Read the model definition and answer for the solid it produces. Units are mm, in the model's axes. A direction names the side the tool comes from. Give positions to 0.01 mm unless a question says otherwise; leave off trailing zeros. Write each loop counter-clockwise with the first axis right and the second up, starting at its lowest first coordinate (ties: lowest second). Pieces come first, ordered by that corner, then holes. Notation, with made-up numbers: (31.25, 66.5) - (44.25, 66.5) arc R13 cw to (44.25, 76.5) - close; hole circle Ø8 at (41, -36.75). An arc over 180 degrees is marked (long way). Answer as CSV lines item,"result".
```python
from build123d import *

# Parameters (mm, degrees)
ESBO_O2_W                = 28
ESBO_O2_H                = 34.43
RESSALTO_EXTRUS_O1_DEPTH = 3
FILETE1_R                = 3
RESSALTO_EXTRUS_O2_START = -1.5
RESSALTO_EXTRUS_O2_DEPTH = 1.5
ESBO_O5_W                = 28
ESBO_O5_H                = 3
RESSALTO_EXTRUS_O3_DEPTH = 20
ESBO_O6_R                = 2.5
CORTE_EXTRUS_O1_DEPTH    = 10
FILETE2_R                = 3
RESSALTO_EXTRUS_O4_DEPTH = 1.5
CHANFRO1_SIZE            = 1.5
CHANFRO2_SIZE            = 1.5
ESBO_O8_R                = 4
CORTE_EXTRUS_O2_DEPTH    = 0.5
CHANFRO3_SIZE            = 5
ESBO_O9_W                = 3
ESBO_O9_H                = 31.43
RESSALTO_EXTRUS_O5_DEPTH = 0.5
CHANFRO4_SIZE            = 0.5


with BuildPart() as part:
    # Esboço2 → Ressalto-extrusão1 (new body)
    with BuildSketch(Plane.XY):
        with Locations((0.050363351, 1.373235294)):
            Rectangle(ESBO_O2_W, ESBO_O2_H)
        with BuildLine():
            Line((8.050363351, 14.888235294), (-7.949636649, 14.888235294))
            ThreePointArc((-7.949636649, 14.888235294), (-9.575982246, 14.214580891), (-10.249636649, 12.588235294))
            Line((-10.249636649, 12.588235294), (-10.249636649, -7.411764706))
            ThreePointArc((-10.249636649, -7.411764706), (-9.575982246, -9.038110303), (-7.949636649, -9.711764706))
            Line((-7.949636649, -9.711764706), (-3.749636649, -9.711764706))
            Line((-3.749636649, -9.711764706), (-3.749636649, -11.711764706))
            Line((-3.749636649, -11.711764706), (3.850363351, -11.711764706))
            Line((3.850363351, -11.711764706), (3.850363351, -9.711764706))
            Line((3.850363351, -9.711764706), (8.050363351, -9.711764706))
            ThreePointArc((8.050363351, -9.711764706), (9.676708947, -9.038110303), (10.350363351, -7.411764706))
            Line((10.350363351, -7.411764706), (10.350363351, 12.588235294))
            ThreePointArc((10.350363351, 12.588235294), (9.676708947, 14.214580891), (8.050363351, 14.888235294))
        make_face(mode=Mode.SUBTRACT)
    extrude(amount=RESSALTO_EXTRUS_O1_DEPTH)

    # Filete1
    filete1_edges = [part.edges().sort_by_distance(p)[0] for p in [
        (-13.949636649, 18.588235294, 1.5),
        (14.050363351, 18.588235294, 1.5),
    ]]
    fillet(filete1_edges, radius=FILETE1_R)

    # Esboço3 → Ressalto-extrusão2 (add)
    with BuildSketch(Plane(origin=(0, 0, 0), x_dir=(-1, 0, 0), z_dir=(0, 0, -1)).offset(RESSALTO_EXTRUS_O2_START)):
        with BuildLine():
            Line((13.949636649, 15.588235294), (13.949636649, -15.841764706))
            Line((13.949636649, -15.841764706), (-14.050363351, -15.841764706))
            Line((-14.050363351, -15.841764706), (-14.050363351, 15.588235294))
            ThreePointArc((-14.050363351, 15.588235294), (-13.171683694, 17.709555638), (-11.050363351, 18.588235294))
            Line((-11.050363351, 18.588235294), (10.949636649, 18.588235294))
            ThreePointArc((10.949636649, 18.588235294), (13.070956993, 17.709555638), (13.949636649, 15.588235294))
        make_face()
    extrude(amount=RESSALTO_EXTRUS_O2_DEPTH)

    # Esboço5 → Ressalto-extrusão3 (add)
    with BuildSketch(Plane(origin=(0, 0, 0), x_dir=(-1, 0, 0), z_dir=(0, 0, -1))):
        with Locations((-0.050363351, -14.341764706)):
            Rectangle(ESBO_O5_W, ESBO_O5_H)
    extrude(amount=RESSALTO_EXTRUS_O3_DEPTH)

    # Esboço6 → Corte-extrusão1 (cut)
    with BuildSketch(Plane(origin=(0, -12.841764706, 0), x_dir=(1, 0, 0), z_dir=(0, 1, 0))):
        with Locations(Location((-7.949636649, 13.5, 0), (0, 0, 180))):
            Circle(ESBO_O6_R)
        with Locations(Location((8.050363351, 13.5, 0), (0, 0, 180))):
            Circle(ESBO_O6_R)
    extrude(amount=-CORTE_EXTRUS_O1_DEPTH, mode=Mode.SUBTRACT)

    # Filete2
    filete2_edges = [part.edges().sort_by_distance(p)[0] for p in [
        (14.050363351, -14.341764706, -20),
        (-13.949636649, -14.341764706, -20),
    ]]
    fillet(filete2_edges, radius=FILETE2_R)

    # Esboço7 → Ressalto-extrusão4 (add, symmetric)
    with BuildSketch(Plane(origin=(0.050363351, 0, 0), x_dir=(0, 0, -1), z_dir=(1, 0, 0))):
        Polygon((0, -1.294759322), (0, -12.841764706), (20, -12.841764706), align=None)
    extrude(amount=RESSALTO_EXTRUS_O4_DEPTH, both=True)

    # Chanfro1
    # the kernel refuses this chamfer: 1.5 mm, written as the material it adds along each edge
    with BuildSketch(Plane(origin=(-1.449636649, -12.841764706, 3.857524482), x_dir=(-0.9996219169112968, -0.027495876610586813, 0), z_dir=(0, 0, -1))) as chanfro1_piece_1_section:
        Polygon((CHANFRO1_SIZE * 0.999621916911, CHANFRO1_SIZE * 0.0274958766106), (-CHANFRO1_SIZE * 0.0274958766106, CHANFRO1_SIZE * 0.999621916911), (0, 0), align=None)
    chanfro1_piece_1 = extrude(amount=27.715048964, mode=Mode.PRIVATE)
    chanfro1_piece_1 = split(chanfro1_piece_1, bisect_by=Plane(origin=(-1.978250847, -8.234905434, -12.020685678), z_dir=(0, -0.8660254037844417, 0.4999999999999947)), keep=Keep.TOP, mode=Mode.PRIVATE)
    chanfro1_piece_1 = split(chanfro1_piece_1, bisect_by=Plane(origin=(-1.978250847, -12.398993102, 1.5), z_dir=(0, 0, -1)), keep=Keep.TOP, mode=Mode.PRIVATE)
    add(chanfro1_piece_1)
    with BuildSketch(Plane(origin=(-1.449636649, 2.56276516, 0), x_dir=(-0.9996219169112969, 0, 0.027495876610586372), z_dir=(0, -1, 0))) as chanfro1_piece_2_section:
        Polygon((CHANFRO1_SIZE * 0.999621916911, CHANFRO1_SIZE * 0.0274958766106), (-CHANFRO1_SIZE * 0.0274958766106, CHANFRO1_SIZE * 0.999621916911), (0, 0), align=None)
    chanfro1_piece_2 = extrude(amount=19.262054348, mode=Mode.PRIVATE)
    chanfro1_piece_2 = split(chanfro1_piece_2, bisect_by=Plane(origin=(-1.952841778, -15.841764706, -0.493589744), z_dir=(0, 1, 0)), keep=Keep.TOP, mode=Mode.PRIVATE)
    chanfro1_piece_2 = split(chanfro1_piece_2, bisect_by=Plane(origin=(-1.952841778, -2.987487395, -2.931891026), z_dir=(0, -0.8660254037844417, 0.4999999999999947)), keep=Keep.TOP, mode=Mode.PRIVATE)
    add(chanfro1_piece_2)
    with BuildSketch(Plane(origin=(1.550363351, -12.841764706, 3.857524482), x_dir=(-0.02749587661058648, 0.9996219169112968, 0), z_dir=(0, 0, -1))) as chanfro1_piece_3_section:
        Polygon((CHANFRO1_SIZE * 0.999621916911, CHANFRO1_SIZE * 0.0274958766106), (-CHANFRO1_SIZE * 0.0274958766106, CHANFRO1_SIZE * 0.999621916911), (0, 0), align=None)
    chanfro1_piece_3 = extrude(amount=27.715048964, mode=Mode.PRIVATE)
    chanfro1_piece_3 = split(chanfro1_piece_3, bisect_by=Plane(origin=(1.674066113, -7.728766139, -11.144026704), z_dir=(0, -0.8660254037844417, 0.4999999999999947)), keep=Keep.TOP, mode=Mode.PRIVATE)
    chanfro1_piece_3 = split(chanfro1_piece_3, bisect_by=Plane(origin=(1.674066113, -11.58917023, 1.5), z_dir=(0, 0, -1)), keep=Keep.TOP, mode=Mode.PRIVATE)
    add(chanfro1_piece_3)
    with BuildSketch(Plane(origin=(1.550363351, 2.56276516, 0), x_dir=(0.9996219169112969, 0, 0.027495876610586372), z_dir=(0, -1, 0))) as chanfro1_piece_4_section:
        Polygon((CHANFRO1_SIZE * 0.999621916911, -CHANFRO1_SIZE * 0.0274958766106), (-CHANFRO1_SIZE * 0.0274958766106, -CHANFRO1_SIZE * 0.999621916911), (0, 0), align=None)
    chanfro1_piece_4 = extrude(amount=15.404529866, mode=Mode.PRIVATE)
    chanfro1_piece_4 = split(chanfro1_piece_4, bisect_by=Plane(origin=(2.053568479, -2.987487395, -2.931891026), z_dir=(0, -0.8660254037844417, 0.4999999999999947)), keep=Keep.TOP, mode=Mode.PRIVATE)
    add(chanfro1_piece_4)

    # Chanfro2
    chanfro2_edges = [part.edges().sort_by_distance(p)[0] for p in [
        (-5.449636649, -12.841764706, -13.5),
        (10.550363351, -12.841764706, -13.5),
    ]]
    chamfer(chanfro2_edges, length=CHANFRO2_SIZE)

    # Esboço8 → Corte-extrusão2 (cut)
    with BuildSketch(Plane.XY.offset(1.5)):
        with Locations((0.050363351, 4.588235294)):
            Circle(ESBO_O8_R)
    extrude(amount=-CORTE_EXTRUS_O2_DEPTH, mode=Mode.SUBTRACT)

    # Chanfro3
    # the kernel refuses this chamfer: 5 mm, written as the material it adds along each edge
    with BuildSketch(Plane(origin=(-13.949636649, -12.841764706, 0), x_dir=(0, -0.027495876610586317, -0.9996219169112968), z_dir=(1, 0, 0))) as chanfro3_piece_1:
        Polygon((CHANFRO3_SIZE * 0.999621916911, CHANFRO3_SIZE * 0.0274958766106), (-CHANFRO3_SIZE * 0.0274958766106, CHANFRO3_SIZE * 0.999621916911), (0, 0), align=None)
    extrude(amount=23.85841494)
    with BuildSketch(Plane(origin=(-9.808051589, -12.841764706, 0), x_dir=(0, 0.9996219169112968, 0.027495876610586372), z_dir=(1, 0, 0))) as chanfro3_piece_2:
        Polygon((CHANFRO3_SIZE * 0.999621916911, -CHANFRO3_SIZE * 0.0274958766106), (-CHANFRO3_SIZE * 0.0274958766106, -CHANFRO3_SIZE * 0.999621916911), (0, 0), align=None)
    extrude(amount=23.85841494)

    # Esboço9 → Ressalto-extrusão5 (add)
    with BuildSketch(Plane(origin=(0, 0, 0), x_dir=(-1, 0, 0), z_dir=(0, 0, -1))):
        with Locations((-8.050363351, 2.873235294)):
            Rectangle(ESBO_O9_W, ESBO_O9_H)
        with Locations((7.949636649, 2.873235294)):
            Rectangle(ESBO_O9_W, ESBO_O9_H)
    extrude(amount=RESSALTO_EXTRUS_O5_DEPTH)

    # Chanfro4
    chanfro4_edges = [part.edges().sort_by_distance(p)[0] for p in [
        (-7.949636649, 18.588235294, -0.5),
        (8.050363351, 18.588235294, -0.5),
    ]]
    chamfer(chanfro4_edges, length=CHANFRO4_SIZE)


solid = part.part
```
(1) A cutting plane is placed at A-A (z = -13.5). Write down the section's boundary in (x, y), and give its area (3 significant figures).
Worked out:
outline,"(-13.95, -15.84) - (-10.45, -15.84) - (-10.45, -14.34) - (-11.95, -12.84) - (-13.95, -12.84) - close; (-5.45, -15.84) - (5.55, -15.84) - (5.55, -14.34) - (4.05, -12.84) - (3.05, -12.84) - (1.55, -11.34) - (1.55, -9.09) - (-1.45, -9.09) - (-1.45, -11.34) - (-2.95, -12.84) - (-3.95, -12.84) - (-5.45, -14.34) - close; (10.55, -15.84) - (14.05, -15.84) - (14.05, -12.84) - (12.05, -12.84) - (10.55, -14.34) - close"
area,"63.0 mm^2"
(2) Each of these flat-tipped pins is pushed along its axis until it touches: P1, Ø6, axis at y = -9.5, z = -15.5, coming from the +X side; P2, Ø5, axis at x = 11, y = 10.5, coming from the -Z side; P3, Ø8, axis at x = -1.5, y = -1.5, coming from the +Z side. Where does it stop, or does it pass through?
Worked out:
P1,"stops at x = 2.71"
P2,"stops at z = -0.5"
P3,"stops at z = 1.5"
(3) For faces 4 (the flat face through (8, 5, -0.5)), 5 (the flat face through (-2.21, -12.1, -11.63)), 6 (the flat face through (10.35, 2, 2)), determine the directions among +Z, -Z, +X, -X, +Y, -Y from which every point of the face is accessible in a straight line to the end or side of a thin tool.
Worked out:
face 4,"-Z, +X, +Y"
face 5,"-Z, -X, +Y"
face 6,"+Z"
(4) A cutting plane is placed at D-D (y = -5.5). Write down the section's boundary in (x, z), and give its area (3 significant figures).
Worked out:
outline,"(-13.95, 0) - (-9.45, 0) - (-9.45, -0.5) - (-6.45, -0.5) - (-6.45, 0) - (-2.95, 0) - (-1.45, -1.5) - (-1.45, -7.28) - (1.55, -7.28) - (1.55, -1.5) - (3.05, 0) - (6.55, 0) - (6.55, -0.5) - (9.55, -0.5) - (9.55, 0) - (14.05, 0) - (14.05, 3) - (10.35, 3) - (10.35, 1.5) - (-10.25, 1.5) - (-10.25, 3) - (-13.95, 3) - close"
area,"80.2 mm^2"
(5) A cutting plane is placed at C-C (x = 0). Write down the section's boundary in (y, z).
Worked out:
outline,"(-15.84, -20) - (-12.84, -20) - (-1.29, 0) - (18.59, 0) - (18.59, 3) - (14.89, 3) - (14.89, 1.5) - (8.59, 1.5) - (8.59, 1) - (0.59, 1) - (0.59, 1.5) - (-11.71, 1.5) - (-11.71, 3) - (-15.84, 3) - close"
(6) The mould has two halves that part along X. Classify faces 1 (the cylindrical face through (-0.817, 0.683, 1.254)), 2 (the flat face through (2.29, -12.08, -11.63)), 3 (the cylindrical face through (-13.09, 17.69, 1.52)): +X half, -X half, draft (parallel to the pull), parting line (faces both ways), or undercut.
Worked out:
face 1,"undercut"
face 2,"+X half"
face 3,"-X half"
(7) A cutting plane is placed at B-B (y = 9.5). Write down the section's boundary in (x, z).
Worked out:
outline,"(-13.95, 0) - (-9.45, 0) - (-9.45, -0.5) - (-6.45, -0.5) - (-6.45, 0) - (6.55, 0) - (6.55, -0.5) - (9.55, -0.5) - (9.55, 0) - (14.05, 0) - (14.05, 3) - (10.35, 3) - (10.35, 1.5) - (-10.25, 1.5) - (-10.25, 3) - (-13.95, 3) - close"
(8) Find the intervals of material crossed by L1, parallel to Z at x = -9.5, y = -2; L2, parallel to Z at x = 10, y = 17; L3, parallel to Y at x = 8.75, z = 2.25, in increasing order.
Worked out:
L1,"z = 0 to 1.5"
L2,"z = 0 to 3"
L3,"y = -15.84 to -9.6, 14.78 to 18.59"
